Build history of the part. All positions in model axes, mm. Give positions to 0.01 mm unless a question says otherwise; leave off trailing zeros. Order: outer loops, then holes, each group sorted by start corner. A loop starts at its lowest first (then second) coordinate and runs counter-clockwise, first axis right, second up. Notation, with made-up numbers: (67.5, 83.5) -> (75.5, 83.5) arc R10 cw to (75.5, 89.5) -> close; hole circle Ø3 at (28.25, -34). An arc over 180 degrees is marked (long way). One line per question, with ' | ' between items. Start each with the question number.
(1) Cut at D-D (y = 17.5). Give the cut face in (x, z), then the cut area to 3 significant figures.
(2) Cut at B-B (y = 193.5). Give the cut face in (x, z).
(3) Cut at C-C (z = 1.6). Give the cut face in (x, y).
(4) Cut at A-A (x = 128.5). Give the cut face in (y, z), then the cut area to 3 significant figures.
(5) Drill centre lines: L1, parallel to X at y = 161, z = 3.75; L2, parallel to Y at x = 129, z = 0.3; L3, parallel to Y at x = 35, z = 0.8. Where is each one in solid material? Low to high. Write a range as from..to.
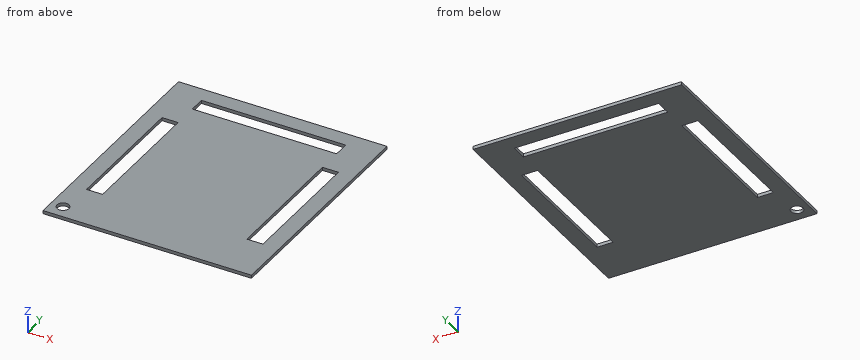
from build123d import *

# Parameters (mm, degrees)
CROQUIS1_W              = 260
CROQUIS1_H              = 296
SALIENTE_EXTRUIR1_DEPTH = 4
CROQUIS2_R              = 7.5
CROQUIS2_W              = 20
CROQUIS2_H              = 165
CROQUIS2_W_2            = 180
CROQUIS2_H_2            = 20
CORTAR_EXTRUIR1_DEPTH   = 4


with BuildPart() as part:
    # Croquis1 → Saliente-Extruir1 (new body)
    with BuildSketch(Plane.XY):
        with Locations((130, 148)):
            Rectangle(CROQUIS1_W, CROQUIS1_H)
    extrude(amount=SALIENTE_EXTRUIR1_DEPTH)

    # Croquis2 → Cortar-Extruir1 (cut)
    with BuildSketch(Plane.XY.offset(4)):
        with Locations((15, 17.5)):
            Circle(CROQUIS2_R)
        with Locations((30, 142.5)):
            Rectangle(CROQUIS2_W, CROQUIS2_H)
        with Locations((230, 142.5)):
            Rectangle(CROQUIS2_W, CROQUIS2_H)
        with Locations((130, 266)):
            Rectangle(CROQUIS2_W_2, CROQUIS2_H_2)
    extrude(amount=-CORTAR_EXTRUIR1_DEPTH, mode=Mode.SUBTRACT)


solid = part.part
Result set:
1) outline: (0, 0) -> (7.5, 0) -> (7.5, 4) -> (0, 4) -> close; (22.5, 0) -> (260, 0) -> (260, 4) -> (22.5, 4) -> close | area: 980 mm2
2) outline: (0, 0) -> (20, 0) -> (20, 4) -> (0, 4) -> close; (40, 0) -> (220, 0) -> (220, 4) -> (40, 4) -> close; (240, 0) -> (260, 0) -> (260, 4) -> (240, 4) -> close
3) outline: (0, 0) -> (260, 0) -> (260, 296) -> (0, 296) -> close; hole circle Ø15 at (15, 17.5); hole (20, 60) -> (40, 60) -> (40, 225) -> (20, 225) -> close; hole (40, 256) -> (220, 256) -> (220, 276) -> (40, 276) -> close; hole (220, 60) -> (240, 60) -> (240, 225) -> (220, 225) -> close
4) outline: (0, 0) -> (256, 0) -> (256, 4) -> (0, 4) -> close; (276, 0) -> (296, 0) -> (296, 4) -> (276, 4) -> close | area: 1,100 mm2
5) L1: x = 0..20, 40..220, 240..260 | L2: y = 0..256, 276..296 | L3: y = 0..60, 225..296
